Verification items for the finished model (mm, model axes). Face numbers are marked on the shaded views. A direction names the side the tool comes from. Coordinates: 2 decimals unless noted, no trailing zeros. Write each loop counter-clockwise with the first axis right and the second up, starting at its lowest first coordinate (ties: lowest second). Pieces come first, ordered by that corner, then holes. Notation, with made-up numbers: (84, -27.5) -> (93, -27.5) arc R22 cw to (93, 10.5) -> close; hole circle Ø9 at (-7.5, 53.25). An arc over 180 degrees is marked (long way). Answer in a Markdown table with one row per item.
```python
from build123d import *

# Parameters (mm, degrees)
SKETCH1_W           = 7.9375
SKETCH1_H           = 15.875
BASE_EXTRUDE_DEPTH  = 19.05
SKETCH2_R           = 2.4384
BOSS_EXTRUDE1_DEPTH = 1.905
LPATTERN6_COUNT     = 2
LPATTERN6_PITCH     = 7.9375
SKETCH4_W           = 4.7625
SKETCH4_H           = 12.7
CUT_EXTRUDE1_DEPTH  = 1.5875
INSDOT_REACH        = 24.757
SKETCH3_R           = 2.032
SKETCH3_R_2         = 1.27
SKETCH5_W           = 6.35
SKETCH5_H           = 13.9065
CUT_EXTRUDE2_DEPTH  = 27.587189144


with BuildPart() as part:
    # Sketch1 → Base-Extrude (new body)
    with BuildSketch(Plane(origin=(0, 0, 0), x_dir=(1, 0, 0), z_dir=(0, 1, 0))):
        Rectangle(SKETCH1_W, SKETCH1_H)
    extrude(amount=BASE_EXTRUDE_DEPTH)

    # Sketch2 → Boss-Extrude1 (add)
    with BuildSketch(Plane(origin=(0, 19.05, 0), x_dir=(-1, 0, 0), z_dir=(0, 1, 0))):
        with Locations(Location((0, 3.96875, 0), (0, 0, 270))):
            Circle(SKETCH2_R)
    boss_extrude1 = extrude(amount=BOSS_EXTRUDE1_DEPTH)

    # LPattern6: Boss-Extrude1 ×2
    with Locations(*[(0, 0, -i * LPATTERN6_PITCH) for i in range(1, LPATTERN6_COUNT)]):
        add(boss_extrude1)

    # Sketch4 → Cut-Extrude1 (cut)
    with BuildSketch(Plane.XZ):
        Rectangle(SKETCH4_W, SKETCH4_H)
    extrude(amount=-CUT_EXTRUDE1_DEPTH, mode=Mode.SUBTRACT)

    # Sketch3 → InsDot (add, up to next)
    with BuildSketch(Plane.XZ, mode=Mode.PRIVATE) as insdot_sk1:
        Circle(SKETCH3_R)
        Circle(SKETCH3_R_2, mode=Mode.SUBTRACT)
    insdot_tool1 = extrude(insdot_sk1.sketch, amount=-INSDOT_REACH, mode=Mode.PRIVATE) - part.part
    add(insdot_tool1.solids().sort_by_distance((-1.974526, 0, 0))[0])

    # Sketch5 → Cut-Extrude2 (cut, through all)
    with BuildSketch(Plane.XY.offset(7.9375)):
        with Locations((0.79375, 10.50925)):
            Rectangle(SKETCH5_W, SKETCH5_H)
    extrude(amount=-CUT_EXTRUDE2_DEPTH, mode=Mode.SUBTRACT)


solid = part.part
```
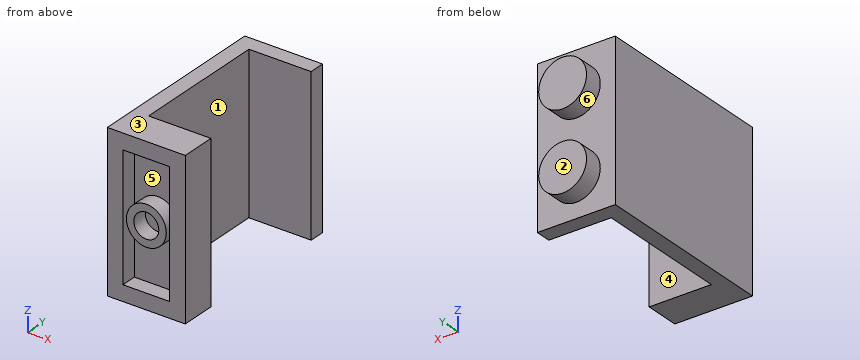
1. Access from +Z, -Z, +X, -X, +Y, -Y to the whole of each face (thin tool, end or side, straight path). Record for the marked faces 4, 5 and 6.
Findings below:
| item | result |
|---|---|
| face 4 | +Z, -Z, +X |
| face 5 | -Y |
| face 6 | +Y |
2. Sectioned sample at B-B, the plane z = 0. Record the cut outline in (x, y).
Findings below:
| item | result |
|---|---|
| outline | (-3.97, 0) -> (-2.38, 0) -> (-2.38, 1.59) -> (-2.03, 1.59) -> (-2.03, 0) -> (-1.27, 0) -> (-1.27, 1.59) -> (1.27, 1.59) -> (1.27, 0) -> (2.03, 0) -> (2.03, 1.59) -> (2.38, 1.59) -> (2.38, 0) -> (3.97, 0) -> (3.97, 3.56) -> (-2.38, 3.56) -> (-2.38, 17.46) -> (3.97, 17.46) -> (3.97, 19.05) -> (-3.97, 19.05) -> close |
3. Material ranges on probe 1 along Z at (x, y) = (0, 1.1); probe 2 along Y at (x, z) = (-1.5, -1); probe 3 along Y at (x, z) = (-0.25, 3.5) (1 decimal), recorded low to high. Write a range as from..to.
Findings below:
| item | result |
|---|---|
| probe 1 | z = -7.94..-6.35, -2.03..-1.27, 1.27..2.03, 6.35..7.94 |
| probe 2 | y = 0..3.56, 17.46..19.05 |
| probe 3 | y = 1.6..3.6, 17.5..21 |
4. Release check for a two-part mould opening along Y. For the marked faces 1, 2 and 3 record: released by +Y, released by -Y, zero draft, split by the parting line, or undercut.
Findings below:
| item | result |
|---|---|
| face 1 | undercut |
| face 2 | released by +Y |
| face 3 | zero draft |
5. Go/stop test with flat-tipped pins: pin 1 (7 mm diameter, centred on y = 13.5, z = 4, fed in from +X); pin 2 (2 mm diameter, centred on x = 0, z = 0, fed in from +Y). Record where each tip stops, or that it passes through.
Findings below:
| item | result |
|---|---|
| pin 1 | stops at x = -2.38 |
| pin 2 | stops at y = 19.05 |
6. Sectioned sample at D-D, the plane y = 10.5. Record the cut outline in (x, z), and give its area (3 significant figures).
Findings below:
| item | result |
|---|---|
| outline | (-3.97, -7.94) -> (-2.38, -7.94) -> (-2.38, 7.94) -> (-3.97, 7.94) -> close |
| area | 25.2 mm² |
7. Sectioned sample at C-C, the plane x = 3.25. Record the cut outline in (y, z), and give its area (3 significant figures).
Findings below:
| item | result |
|---|---|
| outline | (0, -7.94) -> (3.56, -7.94) -> (3.56, 7.94) -> (0, 7.94) -> close; (17.46, -7.94) -> (19.05, -7.94) -> (19.05, 7.94) -> (17.46, 7.94) -> close |
| area | 81.7 mm² |
